Here's how the part is built. I have some questions about the finished solid (model axes, mm). Round coordinates to 2 decimals unless told otherwise and drop trailing zeros. Loops run counter-clockwise (first coordinate to the right, second up) from the corner with the lowest first, then second, coordinate; pieces in that order, holes last. Notation, with made-up numbers: M -39.5,14 L -15.5,14 A14 ccw -15.5,34 Z; hole C 47.5,47.5 d11. An arc over 180 degrees is marked long. Put each result on its own line as item: value. Start each with the question number.
```python
from build123d import *

# Parameters (mm, degrees)
SKETCH1_R                            = 12.7
SKETCH1_R_2                          = 10.7
EXTRUDE_THIN1_DEPTH                  = 2000
SKETCH6_R                            = 12.7
SKETCH6_R_2                          = 10.7
EXTRUDE_THIN4_DEPTH                  = 75
EXTRUDE_THIN5_REACH                  = 2086.148
EXTRUDE_THIN5_END_RADIUS             = 12.7
EXTRUDE_THIN5_START                  = 50
SKETCH7_R                            = 12.7
SKETCH7_R_2                          = 10.7
EXTRUDE_THIN5_DIRECTION_2_REACH      = 2086.148
EXTRUDE_THIN5_DIRECTION_2_END_RADIUS = 12.7
SKETCH8_R                            = 12.7
SKETCH8_R_2                          = 10.7
EXTRUDE_THIN6_DEPTH                  = 75
EXTRUDE_THIN8_REACH                  = 2086.148
EXTRUDE_THIN8_END_RADIUS             = 12.7
EXTRUDE_THIN8_START                  = -50
SKETCH9_R                            = 12.7
SKETCH9_R_2                          = 10.7
EXTRUDE_THIN8_DIRECTION_2_REACH      = 2086.148
EXTRUDE_THIN8_DIRECTION_2_END_RADIUS = 12.7


with BuildPart() as part:
    # Sketch1 → Extrude-Thin1 (new body)
    with BuildSketch(Plane(origin=(0, 0, 0), x_dir=(1, 0, 0), z_dir=(0, 1, 0))):
        Circle(SKETCH1_R)
        Circle(SKETCH1_R_2, mode=Mode.SUBTRACT)
    extrude(amount=EXTRUDE_THIN1_DEPTH)



with BuildPart() as body_2:
    # Sketch6 → Extrude-Thin4 (new, symmetric)
    with BuildSketch(Plane.XY):
        with Locations((350.8, 12.7)):
            Circle(SKETCH6_R)
        with Locations((350.8, 12.7)):
            Circle(SKETCH6_R_2, mode=Mode.SUBTRACT)
    extrude(amount=EXTRUDE_THIN4_DEPTH, both=True)


with BuildPart() as part_1:
    add(part.part)

    add(body_2.part)  # Extrude-Thin5 merges body 2
    # Extrude-Thin5: up to this cylinder (the profile starts outside it)
    extrude_thin5_end = Plane(origin=(350.8, 12.7, 12.34079), z_dir=(0, 0, -1)) * Cylinder(EXTRUDE_THIN5_END_RADIUS, 4198.696, mode=Mode.PRIVATE)
    # Sketch7 → Extrude-Thin5 (add, up to the surface)
    with BuildSketch(Plane(origin=(0, 0, 0), x_dir=(0, 0, -1), z_dir=(1, 0, 0)).offset(EXTRUDE_THIN5_START), mode=Mode.PRIVATE) as extrude_thin5_sk1:
        with Locations((0, 12.7)):
            Circle(SKETCH7_R)
        with Locations((0, 12.7)):
            Circle(SKETCH7_R_2, mode=Mode.SUBTRACT)
    extrude_thin5_tool1 = extrude(extrude_thin5_sk1.sketch, amount=EXTRUDE_THIN5_REACH, mode=Mode.PRIVATE) - extrude_thin5_end
    add(extrude_thin5_tool1.solids().sort_by_distance((50, 12.7, 12.34079))[0])

    # Extrude-Thin5 direction 2: up to this cylinder (the profile starts outside it)
    extrude_thin5_direction_2_end = Plane(origin=(0, 12.7, 0), z_dir=(0, -1, 0)) * Cylinder(EXTRUDE_THIN5_DIRECTION_2_END_RADIUS, 4198.696, mode=Mode.PRIVATE)
    # Sketch7 → Extrude-Thin5 direction 2 (add, up to the surface)
    with BuildSketch(Plane(origin=(0, 0, 0), x_dir=(0, 0, -1), z_dir=(1, 0, 0)).offset(EXTRUDE_THIN5_START), mode=Mode.PRIVATE) as extrude_thin5_direction_2_sk1:
        with Locations((0, 12.7)):
            Circle(SKETCH7_R)
        with Locations((0, 12.7)):
            Circle(SKETCH7_R_2, mode=Mode.SUBTRACT)
    extrude_thin5_direction_2_tool1 = extrude(extrude_thin5_direction_2_sk1.sketch, amount=-EXTRUDE_THIN5_DIRECTION_2_REACH, mode=Mode.PRIVATE) - extrude_thin5_direction_2_end
    add(extrude_thin5_direction_2_tool1.solids().sort_by_distance((50, 12.7, 12.34079))[0])



with BuildPart() as body_2_2:
    # Sketch8 → Extrude-Thin6 (new, symmetric)
    with BuildSketch(Plane.XY):
        with Locations((-350.8, 12.7)):
            Circle(SKETCH8_R)
        with Locations((-350.8, 12.7)):
            Circle(SKETCH8_R_2, mode=Mode.SUBTRACT)
    extrude(amount=EXTRUDE_THIN6_DEPTH, both=True)


with BuildPart() as part_2:
    add(part_1.part)

    add(body_2_2.part)  # Extrude-Thin8 merges body 2 2
    # Extrude-Thin8: up to this cylinder (the profile starts outside it)
    extrude_thin8_end = Plane(origin=(-350.8, 12.7, 12.34079), z_dir=(0, 0, -1)) * Cylinder(EXTRUDE_THIN8_END_RADIUS, 4198.696, mode=Mode.PRIVATE)
    # Sketch9 → Extrude-Thin8 (add, up to the surface)
    with BuildSketch(Plane(origin=(0, 0, 0), x_dir=(0, 0, -1), z_dir=(1, 0, 0)).offset(EXTRUDE_THIN8_START), mode=Mode.PRIVATE) as extrude_thin8_sk1:
        with Locations((0, 12.7)):
            Circle(SKETCH9_R)
        with Locations((0, 12.7)):
            Circle(SKETCH9_R_2, mode=Mode.SUBTRACT)
    extrude_thin8_tool1 = extrude(extrude_thin8_sk1.sketch, amount=-EXTRUDE_THIN8_REACH, mode=Mode.PRIVATE) - extrude_thin8_end
    add(extrude_thin8_tool1.solids().sort_by_distance((-50, 12.7, 12.34079))[0])

    # Extrude-Thin8 direction 2: up to this cylinder (the profile starts outside it)
    extrude_thin8_direction_2_end = Plane(origin=(0, 12.7, 0), z_dir=(0, -1, 0)) * Cylinder(EXTRUDE_THIN8_DIRECTION_2_END_RADIUS, 4198.696, mode=Mode.PRIVATE)
    # Sketch9 → Extrude-Thin8 direction 2 (add, up to the surface)
    with BuildSketch(Plane(origin=(0, 0, 0), x_dir=(0, 0, -1), z_dir=(1, 0, 0)).offset(EXTRUDE_THIN8_START), mode=Mode.PRIVATE) as extrude_thin8_direction_2_sk1:
        with Locations((0, 12.7)):
            Circle(SKETCH9_R)
        with Locations((0, 12.7)):
            Circle(SKETCH9_R_2, mode=Mode.SUBTRACT)
    extrude_thin8_direction_2_tool1 = extrude(extrude_thin8_direction_2_sk1.sketch, amount=EXTRUDE_THIN8_DIRECTION_2_REACH, mode=Mode.PRIVATE) - extrude_thin8_direction_2_end
    add(extrude_thin8_direction_2_tool1.solids().sort_by_distance((-50, 12.7, 12.34079))[0])

    # SurfaceCut1
    split(bisect_by=Plane(origin=(0, 993.65, -993.65), x_dir=(0, -0.7071067811865457, -0.7071067811865493), z_dir=(0, -0.7071067811865493, 0.7071067811865457)), keep=Keep.TOP)


solid = part_2.part
```
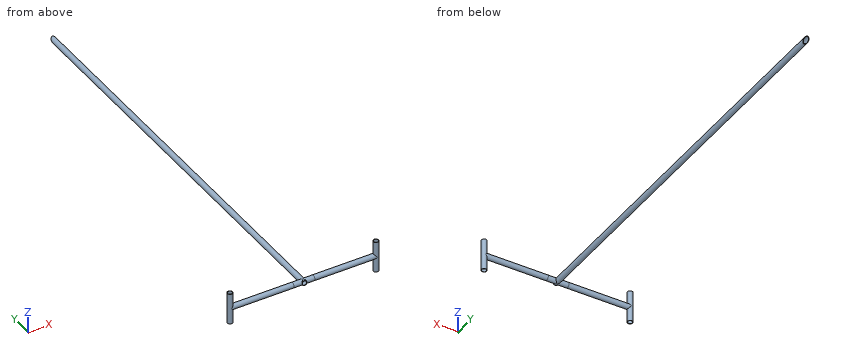
1) Suppose I cut it at B-B (x = -225.5). Write out the boundary of the cut face in (y, z).
2) Suppose I cut it at A-A (z = -33). Write out the boundary of the cut face in (x, y), plus the area to 3 significant figures.
3) Suppose I cut it at C-C (y = 266.5). Write out the boundary of the cut face in (x, z), plus the area to 3 significant figures.
4) If I drill on probe 1 along Z at (x, y) = (30.5, 12.7); probe 2 along Y at (x, z) = (189, 0), over which ranges is the centre line in solid material (lowest first)? Write a range as from..to.
5) I'm going to push a flat-ended pin straight in: P1, Ø4, axis at y = 1159.5, z = 9, coming from the -X side. Where does the tip first touch, or does it pass through?
Results are:
1. outline: C 12.7,0 d25.4; hole C 12.7,0 d21.4
2. outline: C -350.8,12.7 d25.4; C 350.8,12.7 d25.4; hole C -350.8,12.7 d21.4; hole C 350.8,12.7 d21.4
2. area: 294 mm²
3. outline: C 0,0 d25.4; hole C 0,0 d21.4
3. area: 147 mm²
4. probe 1: -12.7..-10.7, 10.7..12.7
4. probe 2: 0..2, 23.4..25.4
5. P1: x = -10.6
